```python
from build123d import *

# Parameters (mm, degrees)
F0_W         = 43
F0_H         = 16
F1_DEPTH     = 6
F2_R         = 2.3
F3_DEPTH     = 16
F2_R_2       = 5.15
F4_DEPTH     = 2.4
F5_R         = 2.3
F6_DEPTH     = 3
F7_T1_DEPTH  = 10
F7_T3_DEPTH  = 41
F7_T5_DEPTH  = 14
F7_S9_W      = 1
F7_S9_H      = 1
F7_T10_DEPTH = 1
F7_S15_W     = 1
F7_S15_H     = 1
F7_T16_DEPTH = 1
F7_S21_W     = 1
F7_S21_H     = 1
F7_T22_DEPTH = 1
F7_S27_W     = 1
F7_S27_H     = 1
F7_T28_DEPTH = 1
F7_S33_W     = 1
F7_S33_H     = 1
F7_T34_DEPTH = 1
F7_S39_W     = 1
F7_S39_H     = 1
F7_T40_DEPTH = 1
F7_S45_W     = 1
F7_S45_H     = 1
F7_T46_DEPTH = 1
F7_S51_W     = 1
F7_S51_H     = 1
F7_T52_DEPTH = 1


# Not quite as in the source:
# - a fillet or chamfer that OpenCascade refuses, or shapes differently, is made with other operations: its cross-section is extruded or revolved along the edge and cut away or added


with BuildPart() as f1:
    # F0 (on Front) → F1 (new body, symmetric)
    with BuildSketch(Plane.XZ):
        Rectangle(F0_W, F0_H)
        with BuildLine():
            ThreePointArc((-7.0434142149, -0.75), (-20, 0), (-7.0434142149, 0.75))
            Line((-7.0434142149, 0.75), (18.5, 0.75))
            Line((18.5, 0.75), (18.5, -0.75))
            Line((18.5, -0.75), (-7.0434142149, -0.75))
        make_face(mode=Mode.SUBTRACT)
    extrude(amount=F1_DEPTH, both=True)

    # F2 (on face) → F3 (cut, through all)
    with BuildSketch(Plane.XY.offset(8)):
        with Locations((11.5, 0)):
            Circle(F2_R)
    extrude(amount=-F3_DEPTH, mode=Mode.SUBTRACT)

    # F2 (on face) → F4 (cut)
    with BuildSketch(Plane.XY.offset(8)):
        with Locations((11.5, 0)):
            Circle(F2_R_2)
        with Locations((11.5, 0)):
            Circle(F2_R, mode=Mode.SUBTRACT)
    extrude(amount=-F4_DEPTH, mode=Mode.SUBTRACT)

    # F5 (on face) → F6 (cut)
    with BuildSketch(Plane(origin=(0, 0, -8), x_dir=(1, 0, 0), z_dir=(0, 0, -1))):
        Polygon((13.5784609691, 3.6), (9.4215390309, 3.6), (7.3430780618, 0), (9.4215390309, -3.6), (13.5784609691, -3.6), (15.6569219382, 0), align=None)
        with Locations((11.5, 0)):
            Circle(F5_R, mode=Mode.SUBTRACT)
    extrude(amount=-F6_DEPTH, mode=Mode.SUBTRACT)

    # F7: fillet of radius 1 on 12 edges, made by hand

    # F7_s2 → F7_t1 (cut)
    with BuildSketch(Plane.XZ.offset(-5)):
        with BuildLine():
            ThreePointArc((-21.5, -7), (-21.2071067812, -7.7071067812), (-20.5, -8))
            Line((-20.5, -8), (-21.5, -8))
            Line((-21.5, -8), (-21.5, -7))
        make_face()
        with BuildLine():
            ThreePointArc((21.5, -7), (21.2071067812, -7.7071067812), (20.5, -8))
            Line((20.5, -8), (21.5, -8))
            Line((21.5, -8), (21.5, -7))
        make_face()
        with BuildLine():
            ThreePointArc((-20.5, 8), (-21.2071067812, 7.7071067812), (-21.5, 7))
            Line((-21.5, 7), (-21.5, 8))
            Line((-21.5, 8), (-20.5, 8))
        make_face()
        with BuildLine():
            ThreePointArc((20.5, 8), (21.2071067812, 7.7071067812), (21.5, 7))
            Line((21.5, 7), (21.5, 8))
            Line((21.5, 8), (20.5, 8))
        make_face()
    extrude(amount=F7_T1_DEPTH, mode=Mode.SUBTRACT)

    # F7_s4 → F7_t3 (cut)
    with BuildSketch(Plane.YZ.offset(-20.5)):
        with BuildLine():
            ThreePointArc((-6, -7), (-5.7071067812, -7.7071067812), (-5, -8))
            Line((-5, -8), (-6, -8))
            Line((-6, -8), (-6, -7))
        make_face()
        with BuildLine():
            ThreePointArc((6, -7), (5.7071067812, -7.7071067812), (5, -8))
            Line((5, -8), (6, -8))
            Line((6, -8), (6, -7))
        make_face()
        with BuildLine():
            ThreePointArc((-5, 8), (-5.7071067812, 7.7071067812), (-6, 7))
            Line((-6, 7), (-6, 8))
            Line((-6, 8), (-5, 8))
        make_face()
        with BuildLine():
            ThreePointArc((5, 8), (5.7071067812, 7.7071067812), (6, 7))
            Line((6, 7), (6, 8))
            Line((6, 8), (5, 8))
        make_face()
    extrude(amount=F7_T3_DEPTH, mode=Mode.SUBTRACT)

    # F7_s6 → F7_t5 (cut)
    with BuildSketch(Plane.XY.offset(-7)):
        with BuildLine():
            ThreePointArc((20.5, 6), (21.2071067812, 5.7071067812), (21.5, 5))
            Line((21.5, 5), (21.5, 6))
            Line((21.5, 6), (20.5, 6))
        make_face()
        with BuildLine():
            ThreePointArc((21.5, -5), (21.2071067812, -5.7071067812), (20.5, -6))
            Line((20.5, -6), (21.5, -6))
            Line((21.5, -6), (21.5, -5))
        make_face()
        with BuildLine():
            ThreePointArc((-20.5, 6), (-21.2071067812, 5.7071067812), (-21.5, 5))
            Line((-21.5, 5), (-21.5, 6))
            Line((-21.5, 6), (-20.5, 6))
        make_face()
        with BuildLine():
            ThreePointArc((-21.5, -5), (-21.2071067812, -5.7071067812), (-20.5, -6))
            Line((-20.5, -6), (-21.5, -6))
            Line((-21.5, -6), (-21.5, -5))
        make_face()
    extrude(amount=F7_T5_DEPTH, mode=Mode.SUBTRACT)


with BuildPart() as f7_tool8:
    # F7_s9 → F7_t10 (new body)
    with BuildSketch(Plane.XZ.offset(-5)):
        with Locations((-21, -7.5)):
            Rectangle(F7_S9_W, F7_S9_H)
    extrude(amount=-F7_T10_DEPTH)

    # F7_s11 → F7_t12 (revolve, cut)
    with BuildSketch(Plane(origin=(-20.5, 5, -7), x_dir=(0.7071067812, 0, 0.7071067812), z_dir=(-0.7071067812, 0, 0.7071067812))):
        with BuildLine():
            ThreePointArc((0, -1), (1, 0), (0, 1))
            Line((0, 1), (0, -1))
        make_face()
    revolve(axis=Axis((-20.5, 5, -7), (0, 1, 0)), mode=Mode.SUBTRACT)


with BuildPart() as f1_1:
    add(f1.part)

    # F7_t7: cut F7_tool8
    add(f7_tool8.part, mode=Mode.SUBTRACT)


with BuildPart() as f7_tool14:
    # F7_s15 → F7_t16 (new body)
    with BuildSketch(Plane.YZ.offset(-20.5)):
        with Locations((-5.5, -7.5)):
            Rectangle(F7_S15_W, F7_S15_H)
    extrude(amount=-F7_T16_DEPTH)

    # F7_s17 → F7_t18 (revolve, cut)
    with BuildSketch(Plane(origin=(-20.5, -5, -7), x_dir=(0, 0.7071067812, 0.7071067812), z_dir=(0, -0.7071067812, 0.7071067812))):
        with BuildLine():
            ThreePointArc((0, -1), (1, 0), (0, 1))
            Line((0, 1), (0, -1))
        make_face()
    revolve(axis=Axis((-20.5, -5, -7), (-1, 0, 0)), mode=Mode.SUBTRACT)


with BuildPart() as f1_2:
    add(f1_1.part)

    # F7_t13: cut F7_tool14
    add(f7_tool14.part, mode=Mode.SUBTRACT)


with BuildPart() as f7_tool20:
    # F7_s21 → F7_t22 (new body)
    with BuildSketch(Plane.YZ.offset(20.5)):
        with Locations((-5.5, -7.5)):
            Rectangle(F7_S21_W, F7_S21_H)
    extrude(amount=F7_T22_DEPTH)

    # F7_s23 → F7_t24 (revolve, cut)
    with BuildSketch(Plane(origin=(20.5, -5, -7), x_dir=(0, 0.7071067812, 0.7071067812), z_dir=(0, 0.7071067812, -0.7071067812))):
        with BuildLine():
            ThreePointArc((0, -1), (1, 0), (0, 1))
            Line((0, 1), (0, -1))
        make_face()
    revolve(axis=Axis((20.5, -5, -7), (1, 0, 0)), mode=Mode.SUBTRACT)


with BuildPart() as f1_3:
    add(f1_2.part)

    # F7_t19: cut F7_tool20
    add(f7_tool20.part, mode=Mode.SUBTRACT)


with BuildPart() as f7_tool26:
    # F7_s27 → F7_t28 (new body)
    with BuildSketch(Plane.XZ.offset(-5)):
        with Locations((21, -7.5)):
            Rectangle(F7_S27_W, F7_S27_H)
    extrude(amount=-F7_T28_DEPTH)

    # F7_s29 → F7_t30 (revolve, cut)
    with BuildSketch(Plane(origin=(20.5, 5, -7), x_dir=(-0.7071067812, 0, 0.7071067812), z_dir=(-0.7071067812, 0, -0.7071067812))):
        with BuildLine():
            ThreePointArc((0, -1), (1, 0), (0, 1))
            Line((0, 1), (0, -1))
        make_face()
    revolve(axis=Axis((20.5, 5, -7), (0, 1, 0)), mode=Mode.SUBTRACT)


with BuildPart() as f1_4:
    add(f1_3.part)

    # F7_t25: cut F7_tool26
    add(f7_tool26.part, mode=Mode.SUBTRACT)


with BuildPart() as f7_tool32:
    # F7_s33 → F7_t34 (new body)
    with BuildSketch(Plane.XY.offset(7)):
        with Locations((21, 5.5)):
            Rectangle(F7_S33_W, F7_S33_H)
    extrude(amount=F7_T34_DEPTH)

    # F7_s35 → F7_t36 (revolve, cut)
    with BuildSketch(Plane(origin=(20.5, 5, 7), x_dir=(-0.7071067812, -0.7071067812, 0), z_dir=(-0.7071067812, 0.7071067812, 0))):
        with BuildLine():
            ThreePointArc((0, -1), (1, 0), (0, 1))
            Line((0, 1), (0, -1))
        make_face()
    revolve(axis=Axis((20.5, 5, 7), (0, 0, 1)), mode=Mode.SUBTRACT)


with BuildPart() as f1_5:
    add(f1_4.part)

    # F7_t31: cut F7_tool32
    add(f7_tool32.part, mode=Mode.SUBTRACT)


with BuildPart() as f7_tool38:
    # F7_s39 → F7_t40 (new body)
    with BuildSketch(Plane.XY.offset(7)):
        with Locations((21, -5.5)):
            Rectangle(F7_S39_W, F7_S39_H)
    extrude(amount=F7_T40_DEPTH)

    # F7_s41 → F7_t42 (revolve, cut)
    with BuildSketch(Plane(origin=(20.5, -5, 7), x_dir=(-0.7071067812, 0.7071067812, 0), z_dir=(0.7071067812, 0.7071067812, 0))):
        with BuildLine():
            ThreePointArc((0, -1), (1, 0), (0, 1))
            Line((0, 1), (0, -1))
        make_face()
    revolve(axis=Axis((20.5, -5, 7), (0, 0, 1)), mode=Mode.SUBTRACT)


with BuildPart() as f1_6:
    add(f1_5.part)

    # F7_t37: cut F7_tool38
    add(f7_tool38.part, mode=Mode.SUBTRACT)


with BuildPart() as f7_tool44:
    # F7_s45 → F7_t46 (new body)
    with BuildSketch(Plane.XY.offset(7)):
        with Locations((-21, 5.5)):
            Rectangle(F7_S45_W, F7_S45_H)
    extrude(amount=F7_T46_DEPTH)

    # F7_s47 → F7_t48 (revolve, cut)
    with BuildSketch(Plane(origin=(-20.5, 5, 7), x_dir=(0.7071067812, -0.7071067812, 0), z_dir=(-0.7071067812, -0.7071067812, 0))):
        with BuildLine():
            ThreePointArc((0, -1), (1, 0), (0, 1))
            Line((0, 1), (0, -1))
        make_face()
    revolve(axis=Axis((-20.5, 5, 7), (0, 0, 1)), mode=Mode.SUBTRACT)


with BuildPart() as f1_7:
    add(f1_6.part)

    # F7_t43: cut F7_tool44
    add(f7_tool44.part, mode=Mode.SUBTRACT)


with BuildPart() as f7_tool50:
    # F7_s51 → F7_t52 (new body)
    with BuildSketch(Plane.XY.offset(7)):
        with Locations((-21, -5.5)):
            Rectangle(F7_S51_W, F7_S51_H)
    extrude(amount=F7_T52_DEPTH)

    # F7_s53 → F7_t54 (revolve, cut)
    with BuildSketch(Plane(origin=(-20.5, -5, 7), x_dir=(0.7071067812, 0.7071067812, 0), z_dir=(0.7071067812, -0.7071067812, 0))):
        with BuildLine():
            ThreePointArc((0, -1), (1, 0), (0, 1))
            Line((0, 1), (0, -1))
        make_face()
    revolve(axis=Axis((-20.5, -5, 7), (0, 0, 1)), mode=Mode.SUBTRACT)


with BuildPart() as f1_8:
    add(f1_7.part)

    # F7_t49: cut F7_tool50
    add(f7_tool50.part, mode=Mode.SUBTRACT)


solid = f1_8.part
```
Part model, mm, in its own coordinate system. A direction names the side the tool comes from. Give positions to 0.01 mm unless a question says otherwise; leave off trailing zeros. Loops run counter-clockwise (first coordinate to the right, second up) from the corner with the lowest first, then second, coordinate; pieces in that order, holes last. Notation, with made-up numbers: M 53,-12.5 L 111,-12.5 A27 cw 111,14.5 Z; hole C -6,64 d1. An arc over 180 degrees is marked long. Return JSON: item names as keys, results as strings.
1) Saw through at A-A, the plane z = 6. List the corners of the cut face in (x, y), then the cut area to 3 significant figures.
Calculated:
{"outline": "M -21.5,-5 A1 ccw -20.5,-6 L -16,-6 L -16,6 L -20.5,6 A1 ccw -21.5,5 Z; M -11,-6 L 20.5,-6 A1 ccw 21.5,-5 L 21.5,5 A1 ccw 20.5,6 L -11,6 Z; hole C 11.5,0 d10.3", "area": "372 mm2"}
2) Pull direction Z, two halves, no side cores. Call faces 1 (the face through (6, 0, -0.75)), 2 (the face through (21.5, 0, 0)), 3 (the face through (-21.199, 0.07, 7.715)): released by +Z, released by -Z, zero draft, split by the parting line, or undercut.
Calculated:
{"face 1": "undercut", "face 2": "zero draft", "face 3": "released by +Z"}
3) 3-axis set-ups, long thin cutter, end or side, ignore diameter. For faces 4 (the face through (14.632, -1.775, -6.521)), 5 (the face through (-20, 0, 0)): which of +Z, -Z, +X, -X, +Y, -Y reach the whole face in a straight line?
Calculated:
{"face 4": "-Z", "face 5": "+Y, -Y"}
4) Saw through at C-C, the plane z = 0. List the corners of the cut face in (x, y).
Calculated:
{"outline": "M -21.5,-5 A1 ccw -20.5,-6 L -20,-6 L -20,6 L -20.5,6 A1 ccw -21.5,5 Z; M 18.5,-6 L 20.5,-6 A1 ccw 21.5,-5 L 21.5,5 A1 ccw 20.5,6 L 18.5,6 Z"}
5) Saw through at D-D, the plane x = 11.5. List the corners of the cut face in (y, z).
Calculated:
{"outline": "M -6,-7 A1 ccw -5,-8 L -3.6,-8 L -3.6,-5 L -2.3,-5 L -2.3,-0.75 L -6,-0.75 Z; M -6,0.75 L -2.3,0.75 L -2.3,5.6 L -5.15,5.6 L -5.15,7.99 A1 ccw -6,7 Z; M 2.3,-5 L 3.6,-5 L 3.6,-8 L 5,-8 A1 ccw 6,-7 L 6,-0.75 L 2.3,-0.75 Z; M 2.3,0.75 L 6,0.75 L 6,7 A1 ccw 5.15,7.99 L 5.15,5.6 L 2.3,5.6 Z"}
6) Saw through at B-B, the plane x = -13.5. List the corners of the cut face in (y, z).
Calculated:
{"outline": "M -6,-7 A1 ccw -5,-8 L 5,-8 A1 ccw 6,-7 L 6,-6.5 L -6,-6.5 Z; M -6,6.5 L 6,6.5 L 6,7 A1 ccw 5,8 L -5,8 A1 ccw -6,7 Z"}
7) Drill centre lines: line 1 (Y direction, x = 11.5, z = -1.8); line 2 (Z direction, x = -3.5, y = 3.75); line 3 (Y direction, x = 11.5, z = 6.3). Where is each one in solid material? Low to high.
Calculated:
{"line 1": "y = -6 to -2.3, 2.3 to 6", "line 2": "z = -8 to -0.75, 0.75 to 8", "line 3": "y = -6 to -5.15, 5.15 to 6"}
8) Flat gauge pin, fed straight in: pin 1 Ø5.5 at (x, y) = (11.5, 0) entering from -Z. Where does the tip first touch, or does it go through?
Calculated:
{"pin 1": "stops at z = -5"}
